from build123d import *


# Not quite as in the source:
# - a feature names something its author has since deleted; it is built from what else it names


with BuildPart() as f1:
    # F0 (on Front) → F1 (revolve)
    with BuildSketch(Plane.XZ):
        with BuildLine():
            Line((-19.9644, 0.412851112), (-20.955, 0.412851112))
            Line((-20.955, 0.412851112), (-20.955, -1.161948888))
            Line((-20.955, -1.161948888), (-19.4564, -1.161948888))
            Line((-19.4564, -1.161948888), (-19.4564, -17.113148888))
            Line((-19.4564, -17.113148888), (-19.0119, -17.113148888))
            ThreePointArc((-19.0119, -17.113148888), (-17.0327575285, -13.4915583263), (-15.8800452648, -9.52870865))
            Line((-15.8800452648, -9.52870865), (-13.5, 3.9691987902))
            ThreePointArc((-13.5, 3.9691987902), (-14.9174256152, 8.8000179565), (-19.4056, 11.080851112))
            Line((-19.4056, 11.080851112), (-19.9644, 11.080851112))
            Line((-19.9644, 11.080851112), (-19.9644, 0.412851112))
        make_face()
    revolve(axis=Axis((0, 0, 12.5831294567), (0, 0, -1)))


solid = f1.part
The model under review builds one solid part; all positions refer to its coordinate system, in mm. A direction names the side the tool comes from. Give positions to 0.01 mm unless a question says otherwise; leave off trailing zeros. Loops run counter-clockwise (first coordinate to the right, second up) from the corner with the lowest first, then second, coordinate; pieces in that order, holes last. Notation, with made-up numbers: (23.5, -6) -> (58.5, -6) arc R22 ccw to (58.5, 14) -> close; hole circle Ø8 at (-21.5, -31.5). An arc over 180 degrees is marked (long way). Write each question's results on one line, items separated by ' | '.
1) Tool access review of faces 1 (the face through (-9, -17, -17.113)), 2 (the face through (8, -19, 0.413)), 3 (the face through (4.218, -18.994, -9.249)): name each direction out of +Z, -Z, +X, -X, +Y, -Y from which nothing blocks a thin tool from reaching the whole face with its end or side.
Conclusion:
face 1: -Z, +X, -X, +Y, -Y | face 2: +Z | face 3: -Z
2) Insertion check: pin 1 Ø2 at (y, z) = (-6.5, 0.5) entering from +X; pin 2 Ø12 at (x, z) = (-8.5, -1) entering from -Y; pin 3 Ø3 at (y, z) = (12.5, 2.5) entering from +X. Each pin has a flat end and moves straight along its axis. Give the tip position at first contact, or say it passes through.
Conclusion:
pin 1: stops at x = 20.22 | pin 2: stops at y = -20.81 | pin 3: stops at x = 16.66
3) For line 1 along Y through (x, z) = (6.5, -7.25); line 2 along X through (y, z) = (6, -10); line 3 along Y through (x, z) = (-13, -11.75), list the stretches that pass through material, from the lowest coordinate up. Write a range as from..to.
Conclusion:
line 1: y = -18.34..-14.05, 14.05..18.34 | line 2: x = -18.51..-14.8, 14.8..18.51 | line 3: y = -14.48..-10.02, 10.02..14.48
4) Take a section at A-A, the plane y = 0. Give the boundary of the cut face in (x, z) (3 decimals).
Conclusion:
outline: (-20.955, -1.162) -> (-19.456, -1.162) -> (-19.456, -17.113) -> (-19.012, -17.113) arc R19.05 ccw to (-15.88, -9.529) -> (-13.5, 3.969) arc R6.35 ccw to (-19.406, 11.081) -> (-19.964, 11.081) -> (-19.964, 0.413) -> (-20.955, 0.413) -> close; (13.5, 3.969) -> (15.88, -9.529) arc R19.05 ccw to (19.012, -17.113) -> (19.456, -17.113) -> (19.456, -1.162) -> (20.955, -1.162) -> (20.955, 0.413) -> (19.964, 0.413) -> (19.964, 11.081) -> (19.406, 11.081) arc R6.35 ccw to start
5) Take a section at C-C, the plane z = -11. Give the boundary of the cut face in (x, y).
Conclusion:
outline: circle Ø38.91 at (0, 0); hole circle Ø32.4 at (0, 0)
6) Draft analysis for pull direction Y (two halves, no side actions). For faces 4 (the face through (2.599, 19.795, 5.672)), 5 (the face through (3.07, -13.81, 0.31)), 6 (the face through (-3.05, 19.32, 11.081)), state which applies: pulls with the +Y half, pulls with the -Y half, needs draft (parallel to the pull), parting line crosses it, or undercut.
Conclusion:
face 4: parting line crosses it | face 5: undercut | face 6: needs draft
7) Take a section at D-D, the plane z = 5.75. Give the boundary of the cut face in (x, y), plus the area to 3 significant figures.
Conclusion:
outline: circle Ø39.93 at (0, 0); hole circle Ø27.07 at (0, 0) | area: 677 mm^2
